from build123d import *

# Parameters (mm, degrees)
F0_R     = 8.5
F0_R_2   = 5.5
F1_DEPTH = 8
F0_R_3   = 3
F2_DEPTH = 8
F3_DEPTH = 6


with BuildPart() as f1:
    # F0 (on Top) → F1 (new body)
    with BuildSketch(Plane.XY):
        Circle(F0_R)
        Circle(F0_R_2, mode=Mode.SUBTRACT)
    extrude(amount=F1_DEPTH)

    # F0 (on Top) → F2 (join)
    with BuildSketch(Plane.XY):
        Circle(F0_R_2)
        Circle(F0_R_3, mode=Mode.SUBTRACT)
    extrude(amount=F2_DEPTH)

    # F0 (on Top) → F3 (cut)
    with BuildSketch(Plane.XY):
        Circle(F0_R_2)
        Circle(F0_R_3, mode=Mode.SUBTRACT)
    extrude(amount=F3_DEPTH, mode=Mode.SUBTRACT)


solid = f1.part
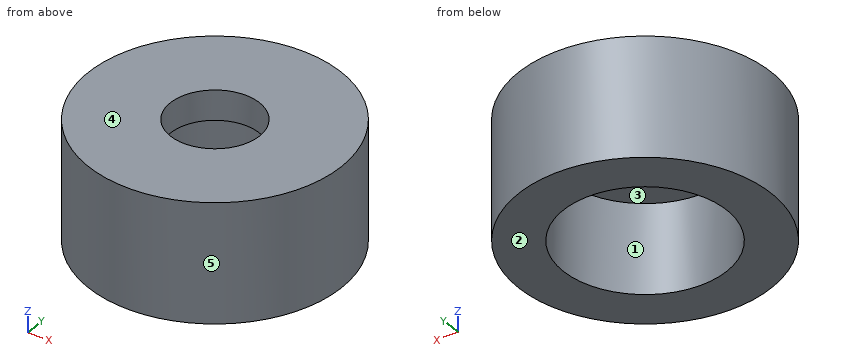
Input: part model. Units: mm. Frame: model coordinates. Face numbers are marked on the shaded views. A direction names the side the tool comes from. Give positions to 0.01 mm unless a question says otherwise; leave off trailing zeros. Order: outer loops, then holes, each group sorted by start corner. A loop starts at its lowest first (then second) coordinate and runs counter-clockwise, first axis right, second up.
Q1. Section A-A on y = 0. Output: boundary loops of the cut face in (x, z).
Checked values:
outline: (-8.5, 0) - (-5.5, 0) - (-5.5, 6) - (-3, 6) - (-3, 8) - (-8.5, 8) - close; (3, 6) - (5.5, 6) - (5.5, 0) - (8.5, 0) - (8.5, 8) - (3, 8) - close
Q2. Contact query for flat-ended pins moving along their axis: pin 1 Ø4 at (x, z) = (7, 6) entering from -Y; pin 2 Ø1 at (x, y) = (3.5, 2.5) entering from -Z; pin 3 Ø8 at (x, y) = (-4, -4.5) entering from -Z; pin 4 Ø2 at (y, z) = (1.5, 3.5) entering from -X. Output: stop coordinate, or through.
Checked values:
pin 1: stops at y = -6.87
pin 2: stops at z = 6
pin 3: stops at z = 0
pin 4: stops at x = -8.49
Q3. Draft query along X for the marked faces 3, 4 and 5. Return one class per face: +X half, -X half, draft (parallel to the pull), parting line (faces both ways), or undercut.
Checked values:
face 3: undercut
face 4: draft
face 5: parting line
Q4. Section C-C on z = 1.5. Output: boundary loops of the cut face in (x, y).
Checked values:
outline: circle Ø17 at (0, 0); hole circle Ø11 at (0, 0)
Q5. Section D-D on x = -4.5. Output: boundary loops of the cut face in (y, z).
Checked values:
outline: (-7.21, 0) - (-3.16, 0) - (-3.16, 6) - (3.16, 6) - (3.16, 0) - (7.21, 0) - (7.21, 8) - (-7.21, 8) - close
Q6. Ray query, probe 1 along Y at (x, z) = (0, 4.1); probe 2 along Y at (x, z) = (0, 7.55); probe 3 along Z at (x, y) = (2.75, -4). Return the intervals inside material, ascending.
Checked values:
probe 1: y = -8.5 to -5.5, 5.5 to 8.5
probe 2: y = -8.5 to -3, 3 to 8.5
probe 3: z = 6 to 8
Q7. Set-up query: the marked faces 1 and 2. Return all of +Z, -Z, +X, -X, +Y, -Y with unobstructed straight access to the full face (end or side cutting, diameter ignored); none if empty.
Checked values:
face 1: -Z
face 2: -Z, +X, -X, +Y, -Y
